```python
from build123d import *

# Parameters (mm, degrees)
CUT_EXTRUDE3_START          = -17
SKETCH4_OUTSIDE_W           = 160.304
SKETCH4_OUTSIDE_H           = 160.304
SKETCH4_OUTSIDE_W_2         = 100
SKETCH4_OUTSIDE_H_2         = 123
CUT_EXTRUDE3_DEPTH          = 17
CUT_EXTRUDE4_REACH          = 86.748
SKETCH5_R                   = 2.5
SKETCH2_R                   = 4
CUT_EXTRUDE5_DEPTH          = 85.748156322
SKETCH6_R                   = 8
CUT_EXTRUDE6_DEPTH          = 13
CHAMFER1_SIZE               = 3
M8_TAPPED_HOLE1_D           = 6.8
M8_TAPPED_HOLE1_DEPTH       = 19.75
M8_TAPPED_HOLE1_CSINK_D     = 8.05
M8_TAPPED_HOLE1_CSINK_ANGLE = 90
M8_TAPPED_HOLE1_TIP         = 2.042926105


with BuildPart() as part:
    # Sketch1 → Revolve1 (revolve)
    with BuildSketch(Plane.XY, mode=Mode.PRIVATE) as revolve1_sk:
        Polygon((42.5, 0), (42.5, 13), (61.5, 13), (61.5, 30), (47.5, 30), (47.5, 22), (0, 22), (0, 0), align=None)
    revolve(revolve1_sk.sketch.rotate(Axis((0, 0, 0), (0, 1, 0)), 90), axis=Axis((0, 0, 0), (0, 1, 0)))

    # Sketch4 outside → Cut-Extrude3 (cut)
    with BuildSketch(Plane(origin=(0, 30, 0), x_dir=(1, 0, 0), z_dir=(0, 1, 0)).offset(CUT_EXTRUDE3_START)):
        Rectangle(SKETCH4_OUTSIDE_W, SKETCH4_OUTSIDE_H)
        Rectangle(SKETCH4_OUTSIDE_W_2, SKETCH4_OUTSIDE_H_2, mode=Mode.SUBTRACT)
    extrude(amount=CUT_EXTRUDE3_DEPTH, mode=Mode.SUBTRACT)

    # Sketch5 → Cut-Extrude4 (cut, up to next)
    with BuildSketch(Plane(origin=(0, 30, 0), x_dir=(1, 0, 0), z_dir=(0, 1, 0)), mode=Mode.PRIVATE) as cut_extrude4_sk1:
        with Locations(Location((-38.183766184, 38.183766184, 0), (0, 0, 270))):
            Circle(SKETCH5_R)
    cut_extrude4_tool1 = extrude(cut_extrude4_sk1.sketch, amount=-CUT_EXTRUDE4_REACH, mode=Mode.PRIVATE) & part.part
    # Sketch5 → Cut-Extrude4 (cut, up to next)
    with BuildSketch(Plane(origin=(0, 30, 0), x_dir=(1, 0, 0), z_dir=(0, 1, 0)), mode=Mode.PRIVATE) as cut_extrude4_sk2:
        with Locations(Location((38.183766184, 38.183766184, 0), (0, 0, 270))):
            Circle(SKETCH5_R)
    cut_extrude4_tool2 = extrude(cut_extrude4_sk2.sketch, amount=-CUT_EXTRUDE4_REACH, mode=Mode.PRIVATE) & part.part
    # Sketch5 → Cut-Extrude4 (cut, up to next)
    with BuildSketch(Plane(origin=(0, 30, 0), x_dir=(1, 0, 0), z_dir=(0, 1, 0)), mode=Mode.PRIVATE) as cut_extrude4_sk3:
        with Locations(Location((38.183766184, -38.183766184, 0), (0, 0, 270))):
            Circle(SKETCH5_R)
    cut_extrude4_tool3 = extrude(cut_extrude4_sk3.sketch, amount=-CUT_EXTRUDE4_REACH, mode=Mode.PRIVATE) & part.part
    # Sketch5 → Cut-Extrude4 (cut, up to next)
    with BuildSketch(Plane(origin=(0, 30, 0), x_dir=(1, 0, 0), z_dir=(0, 1, 0)), mode=Mode.PRIVATE) as cut_extrude4_sk4:
        with Locations(Location((-38.183766184, -38.183766184, 0), (0, 0, 270))):
            Circle(SKETCH5_R)
    cut_extrude4_tool4 = extrude(cut_extrude4_sk4.sketch, amount=-CUT_EXTRUDE4_REACH, mode=Mode.PRIVATE) & part.part
    add(cut_extrude4_tool1.solids().sort_by_distance((-38.183766, 30, -38.183766))[0], mode=Mode.SUBTRACT)
    add(cut_extrude4_tool2.solids().sort_by_distance((38.183766, 30, -38.183766))[0], mode=Mode.SUBTRACT)
    add(cut_extrude4_tool3.solids().sort_by_distance((38.183766, 30, 38.183766))[0], mode=Mode.SUBTRACT)
    add(cut_extrude4_tool4.solids().sort_by_distance((-38.183766, 30, 38.183766))[0], mode=Mode.SUBTRACT)

    # Sketch2 → Cut-Extrude5 (cut, through all)
    with BuildSketch(Plane.XZ):
        with Locations(Location((30, 0, 0), (0, 0, 270))):
            Circle(SKETCH2_R)
        with Locations(Location((0, -30, 0), (0, 0, 270))):
            Circle(SKETCH2_R)
        with Locations(Location((-30, 0, 0), (0, 0, 270))):
            Circle(SKETCH2_R)
        with Locations(Location((0, 30, 0), (0, 0, 270))):
            Circle(SKETCH2_R)
    extrude(amount=-CUT_EXTRUDE5_DEPTH, mode=Mode.SUBTRACT)

    # Sketch6 → Cut-Extrude6 (cut)
    with BuildSketch(Plane.XZ):
        with Locations(Location((0, 30, 0), (0, 0, 270))):
            Circle(SKETCH6_R)
        with Locations(Location((30, 0, 0), (0, 0, 270))):
            Circle(SKETCH6_R)
        with Locations(Location((-30, 0, 0), (0, 0, 270))):
            Circle(SKETCH6_R)
        with Locations(Location((0, -30, 0), (0, 0, 270))):
            Circle(SKETCH6_R)
    extrude(amount=-CUT_EXTRUDE6_DEPTH, mode=Mode.SUBTRACT)

    # Chamfer1
    chamfer1_edges = [part.edges().sort_by_distance(p)[0] for p in [
        (0, 0, 42.5),
    ]]
    chamfer(chamfer1_edges, length=CHAMFER1_SIZE)

    # M8 Tapped Hole1
    with Locations(Plane(origin=(38.183766184, 13, -38.183766184), x_dir=(0, 0, -1), z_dir=(0, -1, 0))):
        with Locations((0, 0), (0, -76.367532368), (-76.367532368, -76.367532368), (-76.367532368, 0)):
            CounterSinkHole(M8_TAPPED_HOLE1_D / 2, M8_TAPPED_HOLE1_CSINK_D / 2, depth=M8_TAPPED_HOLE1_DEPTH, counter_sink_angle=M8_TAPPED_HOLE1_CSINK_ANGLE)
            with Locations((0, 0, -(M8_TAPPED_HOLE1_DEPTH + M8_TAPPED_HOLE1_TIP / 2))):  # 118° drill point
                Cone(0, M8_TAPPED_HOLE1_D / 2, M8_TAPPED_HOLE1_TIP, mode=Mode.SUBTRACT)


solid = part.part
```
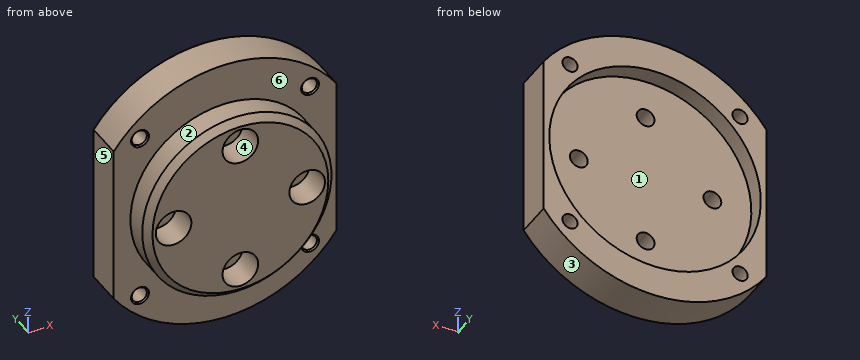
Model file for the job. Use its own axes, mm. Face numbers are marked on the shaded views. A direction names the side the tool comes from. Give positions to 0.01 mm unless a question says otherwise; leave off trailing zeros. Write each loop counter-clockwise with the first axis right and the second up, starting at its lowest first coordinate (ties: lowest second). Pieces come first, ordered by that corner, then holes. Notation, with made-up numbers: (-15.75, 89.25) - (33.25, 89.25) arc R32 ccw to (33.25, 124.25) - close; hole circle Ø8 at (-24.5, -18.75). An arc over 180 degrees is marked (long way). One line per question, with ' | ' between items. Start each with the question number.
(1) Wall check: line 1 along Z through (x, y) = (-6, 2.75); line 2 along Z through (x, y) = (-5.5, 2.25); line 3 along X through (y, z) = (20, -30). Give the ranges that are in metal, low to high. Write a range as from..to.
(2) Pin check, flat tips, straight feed: P1, Ø5.5, axis at x = -38.18, z = -38.18, coming from the +Y side; P2, Ø6, axis at x = 28.5, y = 4.5, coming from the +Z side; P3, Ø8, axis at x = 28.5, y = 9.5, coming from the +Z side; P4, Ø1, axis at x = 34, y = 5, coming from the +Z side. Stop position of each tip, or through.
(3) 3-axis set-ups, long thin cutter, end or side, ignore diameter. For the marked faces 1, 2 and 3: which of +Z, -Z, +X, -X, +Y, -Y reach the whole face in a straight line?
(4) Two-plate mould, pull along X, no slides. Class the marked faces 4, 5 and 6: +X half, -X half, draft (parallel to the pull), parting line (faces both ways), or undercut.
(5) Slice it at A-A on x = 0. Give the number of separate pieces and of enclosed holes in the cut face, plus the area to 3 significant figures.
(6) Slice it at C-C on y = 27.5. Write the cut outline in (x, z).
(7) Slice it at B-B on y = 10.25. Write the cut outline in (x, z), plus the area to 3 significant figures.
Results below:
1) line 1: -41.82..-35.29, -24.71..24.71, 35.29..41.82 | line 2: -41.39..-35.81, -24.19..24.19, 35.81..41.39 | line 3: -50..-4, 4..50
2) P1: through | P2: z = 34 | P3: z = 55.47 | P4: z = 26.15
3) face 1: +Y | face 2: -Y | face 3: -Z, +Y, -Y
4) face 4: undercut | face 5: -X half | face 6: draft
5) separate pieces: 3 | enclosed holes: 0 | area: 1,870 mm^2
6) outline: (-50, -35.81) arc R61.5 ccw to (50, -35.81) - (50, 35.81) arc R61.5 ccw to (-50, 35.81) - close; hole circle Ø95 at (0, 0); hole circle Ø6.8 at (-38.18, -38.18); hole circle Ø6.8 at (-38.18, 38.18); hole circle Ø6.8 at (38.18, -38.18); hole circle Ø6.8 at (38.18, 38.18)
7) outline: circle Ø85 at (0, 0); hole circle Ø16 at (-30, 0); hole circle Ø16 at (0, -30); hole circle Ø16 at (0, 30); hole circle Ø16 at (30, 0) | area: 4,870 mm^2
